Study the drawing (mm; zero at the part's minimum x, y, z) and answer. A direction names the side the tool comes from. Round coordinates to 2 decimals unless told otherwise and drop trailing zeros. Order: outer loops, then holes, each group sorted by start corner. A loop starts at its lowest first (then second) coordinate and runs counter-clockwise, first axis right, second up. Notation, with made-up numbers: (54.25, 76) - (70.25, 76) arc R22 cw to (70.25, 92) - close; hole circle Ø7 at (37.25, 6). An arc over 180 degrees is marked (long way). Use one line per item in the form item = value. Start each with the question number.
Q1. The part is cut by section A-A on z = 34.29. Determine the outline of the cut face in (x, y).
Q2. The part is cut by section D-D on y = 18. Determine the outline of the cut face in (x, z), plus the area to 3 significant figures.
Q3. Which of the six approach directions +Z, -Z, +X, -X, +Y, -Y give full straight-line access (tool end or side, diameter ignored) to the marked faces 1, 2, 3, 4 and 5?
Q4. The part is cut by section C-C on x = 11.5. Determine the outline of the cut face in (y, z).
Q5. The part is cut by section B-B on x = 27.94. Determine the outline of the cut face in (y, z).
Q6. Given P1, Ø2, axis at x = 17, y = 15.5, coming from the -Z side; P2, Ø2, axis at y = 11, z = 24, coming from the +X side; P3, Ø12, axis at y = 10.5, z = 13.5, coming from the -X side; P4, Ø4.5, axis at x = 27.94, z = 3.81, coming from the +Y side, each flat-ended and moving along its own axis, determine where each tip first touches the part or whether it passes through.
Q7. Find the intervals of material crossed by line 1 (X direction, y = 30.3, z = 34.29); line 2 (X direction, y = 30, z = 3); line 3 (Z direction, x = 27, y = 30), in increasing order. Write a range as [from, to].
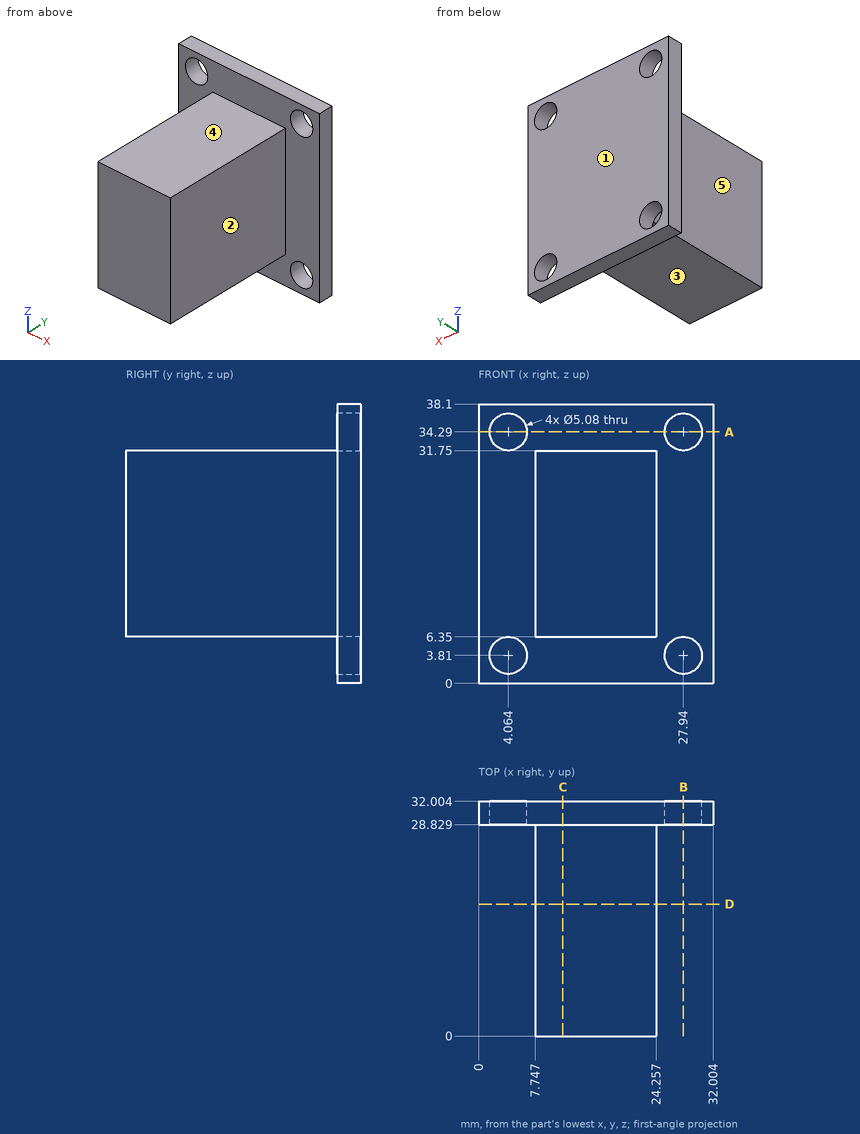
Found:
q1.outline = (0, 28.83) - (1.52, 28.83) - (1.52, 32) - (0, 32) - close; (6.6, 28.83) - (25.4, 28.83) - (25.4, 32) - (6.6, 32) - close; (30.48, 28.83) - (32, 28.83) - (32, 32) - (30.48, 32) - close
q2.outline = (7.75, 6.35) - (24.26, 6.35) - (24.26, 31.75) - (7.75, 31.75) - close
q2.area = 419 mm²
q3.face_1 = +Z, -Z, +X, -X, +Y
q3.face_2 = +Z, -Z, +X, -Y
q3.face_3 = -Z, +X, -X, -Y
q3.face_4 = +Z, +X, -X, -Y
q3.face_5 = +Z, -Z, -X, -Y
q4.outline = (0, 6.35) - (28.83, 6.35) - (28.83, 0) - (32, 0) - (32, 38.1) - (28.83, 38.1) - (28.83, 31.75) - (0, 31.75) - close
q5.outline = (28.83, 0) - (32, 0) - (32, 1.27) - (28.83, 1.27) - close; (28.83, 6.35) - (32, 6.35) - (32, 31.75) - (28.83, 31.75) - close; (28.83, 36.83) - (32, 36.83) - (32, 38.1) - (28.83, 38.1) - close
q6.P1 = 6.35
q6.P2 = 24.26
q6.P3 = 7.75
q6.P4 = through
q7.line_1 = [0, 1.52], [6.6, 25.4], [30.48, 32]
q7.line_2 = [0, 1.66], [6.47, 25.53], [30.35, 32]
q7.line_3 = [0, 1.45], [6.17, 31.93], [36.65, 38.1]
